Geometry check sheet. Reference: the model listing, model coordinates, mm. Face numbers are marked on the shaded views. Give positions to 0.01 mm unless a question says otherwise; leave off trailing zeros. Loops run counter-clockwise (first coordinate to the right, second up) from the corner with the lowest first, then second, coordinate; pieces in that order, holes last. Notation, with made-up numbers: (25.5, 77.25) -> (41.5, 77.25) arc R7 cw to (41.5, 83.25) -> close; hole circle Ø2 at (-11.5, 29). An arc over 180 degrees is marked (long way). One line per item, written item: value. Start each with the question number.
(1) Sectioned sample at A-A, the plane x = 0. Record the cut outline in (y, z), then the cut area to 3 significant figures.
(2) Sectioned sample at B-B, the plane z = 0. Record the cut outline in (x, y), then the cut area to 3 significant figures.
(3) Sectioned sample at C-C, the plane y = 21.5. Record the cut outline in (x, z).
(4) Scan lines: line 1 along X through (y, z) = (-4.5, 0); line 2 along Y through (x, z) = (-1.5, 1); line 3 along Z through (x, y) = (-5, -6.5). Record each from-to range of solid material in increasing order. Write a range as from..to.
(5) Sectioned sample at D-D, the plane y = 5. Record the cut outline in (x, z).
(6) Gauge pin test, flat ends, axial feed: pin 1 Ø4 at (y, z) = (23, -1.5) entering from +X; pin 2 Ø8 at (x, y) = (8, 6.5) entering from -Z; pin 3 Ø12 at (y, z) = (19, 9.5) entering from +X; pin 4 Ø5.5 at (x, z) = (-0.5, 1) entering from -Y. Record the tip position at first contact, or that the pin passes through.
(7) Draft check along Z on the marked faces 1, 2 and 3. Enter one of: pulls with the +Z half, pulls with the -Z half, needs draft (parallel to the pull), parting line crosses it, or undercut.
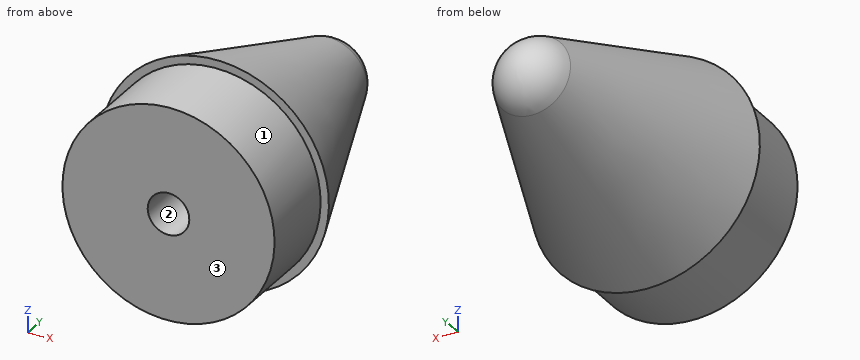
from build123d import *

# Parameters (mm, degrees)
SKETCH6_R           = 12.75
SKETCH6_R_2         = 2.5
BOSS_EXTRUDE2_DEPTH = 10


with BuildPart() as part:
    # Sketch5 → Revolve2 (revolve)
    with BuildSketch(Plane.XY, mode=Mode.PRIVATE) as revolve2_sk:
        with BuildLine():
            Line((0, 0), (-13.75, 0))
            Line((-13.75, 0), (-4.661495631, 24.7))
            ThreePointArc((-4.661495631, 24.7), (-2.841825215, 27.058541596), (0, 27.951821134))
            Line((0, 27.951821134), (0, 24.7))
            Line((0, 24.7), (0, 0))
        make_face()
    revolve(revolve2_sk.sketch.rotate(Axis((0, 0, 0), (0, 1, 0)), 270), axis=Axis((0, 0, 0), (0, 1, 0)))

    # Sketch6 → Boss-Extrude2 (add)
    with BuildSketch(Plane.XZ):
        with Locations(Location((0, 0, 0), (0, 0, 90))):
            Circle(SKETCH6_R)
        with Locations(Location((0, 0, 0), (0, 0, 270))):
            Circle(SKETCH6_R_2, mode=Mode.SUBTRACT)
    extrude(amount=BOSS_EXTRUDE2_DEPTH)


solid = part.part
Calculated:
1. outline: (-10, -12.75) -> (0, -12.75) -> (0, -13.75) -> (24.7, -4.66) arc R4.97 ccw to (24.7, 4.66) -> (0, 13.75) -> (0, 12.75) -> (-10, 12.75) -> (-10, 2.5) -> (0, 2.5) -> (0, -2.5) -> (-10, -2.5) -> close
1. area: 682 mm2
2. outline: (-13.75, 0) -> (-12.75, 0) -> (-12.75, -10) -> (-2.5, -10) -> (-2.5, 0) -> (2.5, 0) -> (2.5, -10) -> (12.75, -10) -> (12.75, 0) -> (13.75, 0) -> (4.66, 24.7) arc R4.97 ccw to (-4.66, 24.7) -> close
2. area: 682 mm2
3. outline: circle Ø11.68 at (0, 0)
4. line 1: x = -12.75..-2.5, 2.5..12.75
4. line 2: y = 0..27.61
4. line 3: z = -11.73..11.73
5. outline: circle Ø23.82 at (0, 0)
6. pin 1: stops at x = 5.92
6. pin 2: stops at z = -11.27
6. pin 3: stops at x = 6.59
6. pin 4: stops at y = -10
7. face 1: parting line crosses it
7. face 2: undercut
7. face 3: needs draft
